Geometry check sheet. Reference: the model listing, model coordinates, mm. Round coordinates to 2 decimals unless told otherwise and drop trailing zeros. Loops run counter-clockwise (first coordinate to the right, second up) from the corner with the lowest first, then second, coordinate; pieces in that order, holes last. Notation, with made-up numbers: M 32.5,44 L 38.5,44 A13 cw 38.5,68 Z; hole C 48,-28 d1. An arc over 180 degrees is marked long. Use one line per item in the form item = value. Start each with the question number.
1. Cross-section at A-A (z = 0). Record the boundary of the cut face in (x, y) (3 decimals), then the cut area to 3 significant figures.
2. Cross-section at B-B (y = 0.25). Record the boundary of the cut face in (x, z).
3. Draft check along Z on faces 1 (the cylindrical face through (158.457, 0.044, 1.907)), 2 (the flat face through (2, 0, 12.7)), 3 (the cylindrical face through (165.097, -0.044, -0.279)). Enter one of: pulls with the +Z half, pulls with the -Z half, needs draft (parallel to the pull), parting line crosses it, or undercut.
4. Material ranges on line 1 (Z direction, x = 152.4, y = -1.25); line 2 (X direction, y = -1.25, z = 5.75); line 3 (X direction, y = 1.75, z = -3.75), recorded low to high.
```python
from build123d import *

# Parameters (mm, degrees)
F0_R     = 6.35
F1_DEPTH = 3.175


with BuildPart() as f1:
    # F0 (on Front) → F1 (new body, symmetric)
    with BuildSketch(Plane.XZ):
        with BuildLine():
            ThreePointArc((152.4, -12.7), (165.1, 0), (152.4, 12.7))
            Line((152.4, 12.7), (-152.4, 12.7))
            Line((-152.4, 12.7), (-152.4, -12.7))
            Line((-152.4, -12.7), (152.4, -12.7))
        make_face()
        with Locations((152.4, 0)):
            Circle(F0_R, mode=Mode.SUBTRACT)
    extrude(amount=F1_DEPTH, both=True)


solid = f1.part
```
Reported:
q1.outline = M -152.4,-3.175 L 146.05,-3.175 L 146.05,3.175 L -152.4,3.175 Z; M 158.75,-3.175 L 165.1,-3.175 L 165.1,3.175 L 158.75,3.175 Z
q1.area = 1,940 mm²
q2.outline = M -152.4,-12.7 L 152.4,-12.7 A12.7 ccw 152.4,12.7 L -152.4,12.7 Z; hole C 152.4,0 d12.7
q3.face_1 = undercut
q3.face_2 = pulls with the +Z half
q3.face_3 = parting line crosses it
q4.line_1 = -12.7 to -6.35, 6.35 to 12.7
q4.line_2 = -152.4 to 149.71, 155.09 to 163.72
q4.line_3 = -152.4 to 147.28, 157.52 to 164.53
